```python
from build123d import *

# Parameters (mm, degrees)
BOSS_EXTRUDE1_DEPTH = 39
SKETCH2_R           = 2.25
BOSS_EXTRUDE2_DEPTH = 24
SKETCH3_R           = 11
BOSS_EXTRUDE3_DEPTH = 2
SKETCH4_R           = 1.5
CUT_EXTRUDE1_DEPTH  = 4.5
CUT_EXTRUDE2_DEPTH  = 15


with BuildPart() as part:
    # Sketch1 → Boss-Extrude1 (new body)
    with BuildSketch(Plane(origin=(0, 0, 0), x_dir=(1, 0, 0), z_dir=(0, 1, 0))):
        Polygon((-21, 18.171572875), (-18.171572875, 21), (18.171572875, 21), (21, 18.171572875), (21, -17), (17, -21), (-18.171572875, -21), (-21, -18.171572875), align=None)
    extrude(amount=BOSS_EXTRUDE1_DEPTH)

    # Sketch2 → Boss-Extrude2 (add)
    with BuildSketch(Plane(origin=(0, 39, 0), x_dir=(1, 0, 0), z_dir=(0, 1, 0))):
        Circle(SKETCH2_R)
    extrude(amount=BOSS_EXTRUDE2_DEPTH)

    # Sketch3 → Boss-Extrude3 (add)
    with BuildSketch(Plane(origin=(0, 39, 0), x_dir=(1, 0, 0), z_dir=(0, 1, 0))):
        Circle(SKETCH3_R)
    extrude(amount=BOSS_EXTRUDE3_DEPTH)

    # Sketch4 → Cut-Extrude1 (cut)
    with BuildSketch(Plane(origin=(0, 39, 0), x_dir=(1, 0, 0), z_dir=(0, 1, 0))):
        with Locations((-15.5, 15.5)):
            Circle(SKETCH4_R)
        with Locations((15.5, 15.5)):
            Circle(SKETCH4_R)
    cut_extrude1 = extrude(amount=-CUT_EXTRUDE1_DEPTH, mode=Mode.SUBTRACT)

    # Mirror1: Cut-Extrude1 across plane
    add(cut_extrude1.mirror(Plane.XY), mode=Mode.SUBTRACT)

    # Sketch5 → Cut-Extrude2 (cut)
    with BuildSketch(Plane(origin=(0, 63, 0), x_dir=(1, 0, 0), z_dir=(0, 1, 0))):
        with BuildLine():
            Line((1.870828693, 1.25), (-1.870828693, 1.25))
            ThreePointArc((-1.870828693, 1.25), (0, 2.25), (1.870828693, 1.25))
        make_face()
    extrude(amount=-CUT_EXTRUDE2_DEPTH, mode=Mode.SUBTRACT)


solid = part.part
```
Source: CAD feature listing. Evaluate the final solid. Frame: model axes, mm. A direction names the side the tool comes from. Coordinates: 2 decimals unless noted, no trailing zeros. Write each loop counter-clockwise with the first axis right and the second up, starting at its lowest first coordinate (ties: lowest second). Pieces come first, ordered by that corner, then holes. Notation, with made-up numbers: M 72.25,23 L 108.25,23 A30 cw 108.25,56 Z; hole C 57,-21 d3. An arc over 180 degrees is marked long. Answer as a JSON object with one key per item and string values.
1. Contact query for flat-ended pins moving along their axis: P1, Ø2.5, axis at x = 15.5, z = -15, coming from the +Y side; P2, Ø4, axis at x = 0, y = 53, coming from the -Z side; P3, Ø5, axis at y = 46.5, z = -6, coming from the +X side; P4, Ø8, axis at x = -5, z = 10, coming from the +Y side. Output: stop coordinate, or through.
Evaluation:
{"P1": "y = 39", "P2": "z = -1.25", "P3": "through", "P4": "y = 41"}
2. Cut plane B-B on x = 0. Output: boundary loops of the cut face in (y, z).
Evaluation:
{"outline": "M 0,-21 L 39,-21 L 39,-11 L 41,-11 L 41,-2.25 L 48,-2.25 L 48,-1.25 L 63,-1.25 L 63,2.25 L 41,2.25 L 41,11 L 39,11 L 39,21 L 0,21 Z"}
3. Ray query, L1, parallel to Z at x = 15.5, y = 36.7; L2, parallel to Z at x = 15, y = 35; L3, parallel to Y at x = -2, z = 15. Return the intervals inside material, ascending.
Evaluation:
{"L1": "-21 to -17, -14 to 14, 17 to 21", "L2": "-21 to -16.91, -14.09 to 14.09, 16.91 to 21", "L3": "0 to 39"}
4. Cut plane C-C on z = 0. Output: boundary loops of the cut face in (x, y), plus the area to 3 significant figures.
Evaluation:
{"outline": "M -21,0 L 21,0 L 21,39 L 11,39 L 11,41 L 2.25,41 L 2.25,63 L -2.25,63 L -2.25,41 L -11,41 L -11,39 L -21,39 Z", "area": "1,780 mm^2"}
5. Access query for faces 5 (the flat face through (-19.606, 19.227, -19.566)), 6 (the flat face through (15, 34.5, -16)), 7 (the flat face through (0, 56, -1.25)). Directions: +Z, -Z, +X, -X, +Y, -Y. A direction counts if a zero-diameter tool reaches every point of the face in a straight line with its end or side. Return the directions, or none.
Evaluation:
{"face 5": "-Z, -X, +Y, -Y", "face 6": "+Y", "face 7": "-Z, +X, -X, +Y"}
6. Cut plane A-A on y = 35.5. Output: boundary loops of the cut face in (x, z), plus the area to 3 significant figures.
Evaluation:
{"outline": "M -21,-18.17 L -18.17,-21 L 18.17,-21 L 21,-18.17 L 21,17 L 17,21 L -18.17,21 L -21,18.17 Z; hole C -15.5,-15.5 d3; hole C -15.5,15.5 d3; hole C 15.5,-15.5 d3; hole C 15.5,15.5 d3", "area": "1,720 mm^2"}
7. Cut plane D-D on z = -15.5. Output: boundary loops of the cut face in (x, y), plus the area to 3 significant figures.
Evaluation:
{"outline": "M -21,0 L 21,0 L 21,39 L 17,39 L 17,34.5 L 14,34.5 L 14,39 L -14,39 L -14,34.5 L -17,34.5 L -17,39 L -21,39 Z", "area": "1,610 mm^2"}
8. Draft query along X for faces 1 (the flat face through (19, 19, 19)), 2 (the cylindrical face through (14, 36.78, -15.57)), 3 (the flat face through (10, 39, 9)), 4 (the flat face through (-16, 34.5, 16)). Return one class per face: released by +X, released by -X, zero draft, split by the parting line, or undercut.
Evaluation:
{"face 1": "released by +X", "face 2": "undercut", "face 3": "zero draft", "face 4": "undercut"}
